Geometry: final body of the model. Coordinates: model frame, mm. A direction names the side the tool comes from. Round coordinates to 2 decimals unless told otherwise and drop trailing zeros. Order: outer loops, then holes, each group sorted by start corner. A loop starts at its lowest first (then second) coordinate and runs counter-clockwise, first axis right, second up. Notation, with made-up numbers: M 49.25,-4 L 74.25,-4 A14 cw 74.25,20 Z; hole C -28.75,-39.75 d6. An arc over 180 degrees is marked long. Put each result on its own line as item: value. Start each with the question number.
1) Draft query along Y for faces 1 (the flat face through (-4, 0, 2)), 2 (the cylindrical face through (-19.296, -19.397, 1.014)), 3 (the flat face through (-27.898, 0, 4)), 4 (the cylindrical face through (-21.93, 11.95, 7.43)). Return one class per face: pulls with the +Y half, pulls with the -Y half, needs draft (parallel to the pull), parting line crosses it, or undercut.
2) Section A-A, the plane x = 1.5. Count the separate pieces of the cut face and the enclosed holes in it, then the cut area to 3 significant figures.
3) Section D-D, the plane x = 9.5. Return loops of the section in (y, z), then the cut area to 3 significant figures.
4) Access query for faces 5 (the flat face through (-4, -10.5, 6)), 6 (the flat face through (-19.898, -15, 1)), 7 (the flat face through (19, -5, 4)), 8 (the flat face through (-1.898, -11, 9)), 9 (the flat face through (0, 15.533, 1)). Directions: +Z, -Z, +X, -X, +Y, -Y. A direction counts if a zero-diameter tool reaches every point of the face in a straight line with its end or side. Return the directions, or none.
5) Material intervals for probe 1 along Y at (x, z) = (16, 8.5); probe 2 along Y at (x, z) = (17, 1); probe 3 along Z at (x, y) = (11.5, -4.5), sorted ascending. Write a range as [from, to].
6) Section C-C, the plane y = -1.5. Return loops of the section in (x, z).
7) First-contact query: P1, Ø1, axis at x = -26.5, z = 7.5, coming from the +Y side; P2, Ø3, axis at x = -12, z = 5, coming from the -Y side; P3, Ø1, axis at y = -14, z = 0.5, coming from the -X side. Flat tips, straight axial feed; report the tip coordinate or a pass-through.
from build123d import *

# Parameters (mm, degrees)
F1_DEPTH     = 2
F2_R         = 2
F3_D         = 3
F7_DEPTH     = 2
F6_W         = 4
F6_H         = 1.95
F6_H_2       = 2.05
F6_H_3       = 2.0331665652
F8_DEPTH     = 8
F6_W_2       = 18
F9_DEPTH     = 10
F10_T1_DEPTH = 4
F10_T3_DEPTH = 4
F11_DEPTH    = 4
F6_W_3       = 2
F6_H_4       = 16
F12_DEPTH    = 6


# Not quite as in the source:
# - a fillet or chamfer that OpenCascade refuses, or shapes differently, is made with other operations: its cross-section is extruded or revolved along the edge and cut away or added


with BuildPart() as f1:
    # F0 (on Top) → F1 (new body)
    with BuildSketch(Plane.XY):
        Polygon((-19.8978664808, -19.9668334348), (0.1021335192, -19.9668334348), (0.1021335192, -15.4668334348), (-1.8978664808, -15.4668334348), (-1.8978664808, -12.4668334348), (0.1021335192, -12.4668334348), (0.1021335192, 0.0331665652), (-19.8978664808, 0.0331665652), align=None)
    extrude(amount=F1_DEPTH)

    # F2
    f2_edges = [f1.edges().sort_by_distance(p)[0] for p in [
        (-19.897866, -19.966833, 1),
    ]]
    fillet(f2_edges, radius=F2_R)

    # F3 (through all)
    with Locations(Plane(origin=(0, 0, 0), x_dir=(1, 0, 0), z_dir=(0, 0, -1))):
        with Locations((-17.3978664808, 17.4668334348)):
            Hole(F3_D / 2)

    # F4: F1 across face


with BuildPart() as f1_1:
    add(f1.part)
    add(f1.part.mirror(Plane(origin=(0.1021335192, -6.2168334348, 1), x_dir=(0, 1, 0), z_dir=(1, 0, 0))))

    # F5: F1 across face


with BuildPart() as f1_2:
    add(f1_1.part)
    add(f1_1.part.mirror(Plane(origin=(0.1021335192, 0.0331665652, 1), x_dir=(-1, 0, 0), z_dir=(0, 1, 0))))

    # F6 (on face) → F7 (join)
    with BuildSketch(Plane(origin=(0, 0, 0), x_dir=(1, 0, 0), z_dir=(0, 0, -1))):
        Polygon((-25.8978664808, -10.5), (-23.8978664808, -10.5), (-19.8978664808, -10.5), (-19.8978664808, 10.5), (-23.8978664808, 10.5), (-25.8978664808, 10.5), (-25.8978664808, 9.5), (-25.8978664808, -6.5), align=None)
        Polygon((18.1021335192, 0), (20.1021335192, -0.05), (20.1021335192, 9.5), (18.1021335192, 9.5), align=None)
        Polygon((-19.8978664808, 10.5), (-19.8978664808, -10.5), (-1.8978664808, -10.5), (2.1021335192, -10.5), (18.1021335192, -10.5), (18.1021335192, 0), (18.1021335192, 9.5), (18.1021335192, 10.5), (2.1021335192, 10.5), (-1.8978664808, 10.5), align=None)
    extrude(amount=-F7_DEPTH)

    # F6 (on face) → F8 (join)
    with BuildSketch(Plane(origin=(0, 0, 0), x_dir=(1, 0, 0), z_dir=(0, 0, -1))):
        with Locations((-21.8978664808, 11.475)):
            Rectangle(F6_W, F6_H)
        with Locations((-21.8978664808, -11.525)):
            Rectangle(F6_W, F6_H_2)
        with Locations((0.1021335192, -11.5165832826)):
            Rectangle(F6_W, F6_H_3)
        with Locations((0.1021335192, 11.475)):
            Rectangle(F6_W, F6_H)
    extrude(amount=-F8_DEPTH)

    # F6 (on face) → F9 (join)
    with BuildSketch(Plane(origin=(0, 0, 0), x_dir=(1, 0, 0), z_dir=(0, 0, -1))):
        Polygon((-27.8978664808, -12.55), (-23.8978664808, -12.55), (-23.8978664808, -10.5), (-25.8978664808, -10.5), (-25.8978664808, -6.5), (-27.8978664808, -6.5), align=None)
        Polygon((-27.8978664808, 12.45), (-27.8978664808, 9.5), (-25.8978664808, 9.5), (-25.8978664808, 10.5), (-23.8978664808, 10.5), (-23.8978664808, 12.45), align=None)
        Polygon((-19.8978664808, -10.5), (-19.8978664808, -12.55), (-1.8978664808, -12.55), (-1.8978664808, -12.5331665652), (-1.8978664808, -10.5), align=None)
        Polygon((2.1021335192, -12.5331665652), (2.1021335192, -12.55), (20.1021335192, -12.55), (20.1021335192, -0.05), (18.1021335192, 0), (18.1021335192, -10.5), (2.1021335192, -10.5), align=None)
        Polygon((2.1021335192, 12.45), (2.1021335192, 10.5), (18.1021335192, 10.5), (18.1021335192, 9.5), (20.1021335192, 9.5), (20.1021335192, 12.45), align=None)
        with Locations((-10.8978664808, 11.475)):
            Rectangle(F6_W_2, F6_H)
    extrude(amount=-F9_DEPTH)

    # F10: fillet of radius 2 on 4 edges, made by hand

    # F10_s2 → F10_t1 (cut)
    with BuildSketch(Plane.YZ.offset(-23.8978664808)):
        with BuildLine():
            ThreePointArc((10.55, 8), (11.9642135624, 7.4142135624), (12.55, 6))
            Line((12.55, 6), (12.55, 8))
            Line((12.55, 8), (10.55, 8))
        make_face()
        with BuildLine():
            ThreePointArc((-12.45, 6), (-11.8642135624, 7.4142135624), (-10.45, 8))
            Line((-10.45, 8), (-12.45, 8))
            Line((-12.45, 8), (-12.45, 6))
        make_face()
    extrude(amount=F10_T1_DEPTH, mode=Mode.SUBTRACT)

    # F10_s4 → F10_t3 (cut)
    with BuildSketch(Plane.YZ.offset(-1.8978664808)):
        with BuildLine():
            ThreePointArc((-12.45, 6), (-11.8642135624, 7.4142135624), (-10.45, 8))
            Line((-10.45, 8), (-12.45, 8))
            Line((-12.45, 8), (-12.45, 6))
        make_face()
        with BuildLine():
            ThreePointArc((12.5331665652, 6), (11.9473801276, 7.4142135624), (10.5331665652, 8))
            Line((10.5331665652, 8), (12.5331665652, 8))
            Line((12.5331665652, 8), (12.5331665652, 6))
        make_face()
    extrude(amount=F10_T3_DEPTH, mode=Mode.SUBTRACT)

    # F6 (on face) → F11 (join)
    with BuildSketch(Plane(origin=(0, 0, 0), x_dir=(1, 0, 0), z_dir=(0, 0, -1))):
        Polygon((18.1021335192, 0), (20.1021335192, -0.05), (20.1021335192, 9.5), (18.1021335192, 9.5), align=None)
    extrude(amount=-F11_DEPTH)

    # F6 (on face) → F12 (join)
    with BuildSketch(Plane(origin=(0, 0, 0), x_dir=(1, 0, 0), z_dir=(0, 0, -1))):
        with Locations((-26.8978664808, 1.5)):
            Rectangle(F6_W_3, F6_H_4)
    extrude(amount=-F12_DEPTH)


solid = f1_2.part
Result sheet:
1. face 1: undercut
1. face 2: pulls with the -Y half
1. face 3: needs draft
1. face 4: pulls with the +Y half
2. separate pieces: 3
2. enclosed holes: 0
2. area: 90.2 mm2
3. outline: M -19.97,0 L 20.03,0 L 20.03,2 L 12.55,2 L 12.55,10 L 10.5,10 L 10.5,2 L -10.5,2 L -10.5,10 L -12.45,10 L -12.45,2 L -19.97,2 Z
3. area: 112 mm2
4. face 5: +Z
4. face 6: +Z, -Z, -X, -Y
4. face 7: +Z, +X
4. face 8: +Z, -Y
4. face 9: +Z, -Z
5. probe 1: y = [-12.45, -10.5], [10.5, 12.55]
5. probe 2: y = [-19.97, -18.84], [-16.09, 16.16], [18.91, 20.03]
5. probe 3: z = [0, 2]
6. outline: M -27.9,0 L 20.1,0 L 20.1,4 L 18.1,4 L 18.1,2 L -25.9,2 L -25.9,6 L -27.9,6 Z
7. P1: stops at y = 12.55
7. P2: stops at y = -12.45
7. P3: stops at x = -19.9
